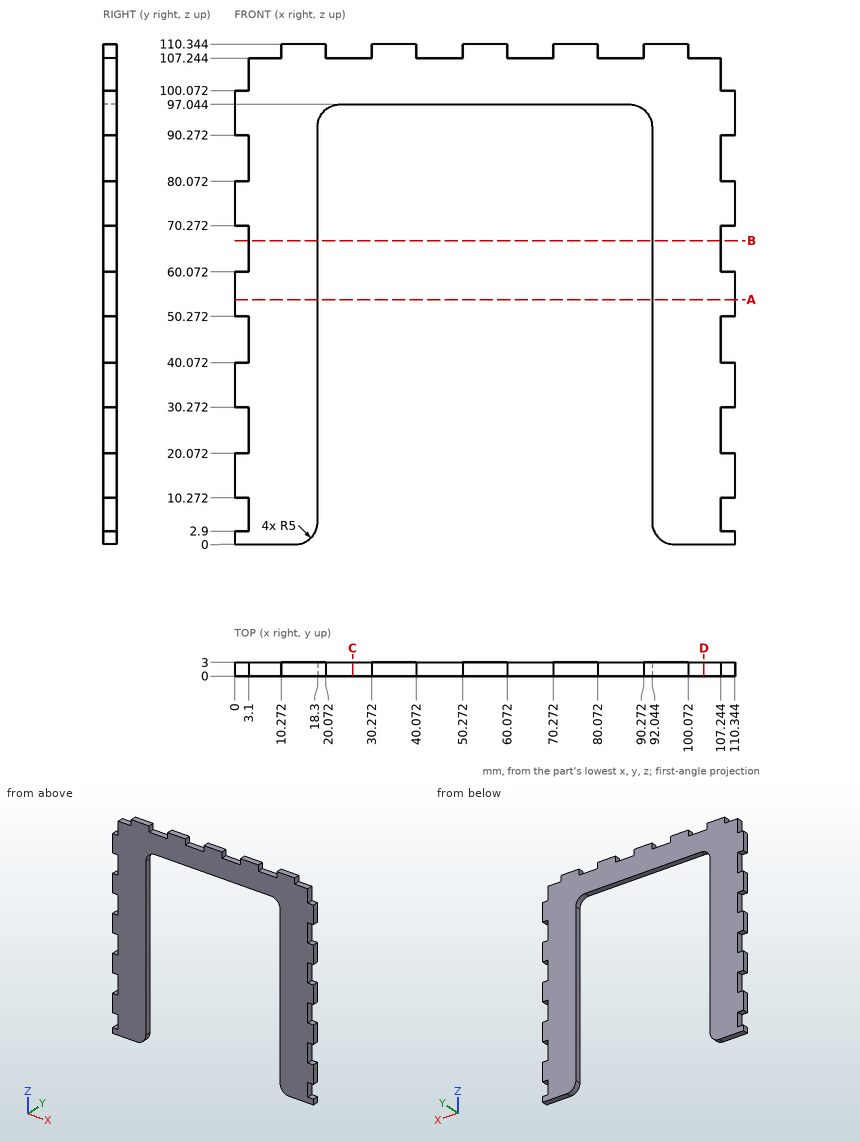
Answer from the drawing. Dimensions are ordinates in mm from the lowest x, y and z of the part. Give positions to 0.01 mm unless a question says otherwise; leave off trailing zeros. Write each loop counter-clockwise with the first axis right and the second up, starting at its lowest first coordinate (ties: lowest second). Pieces come first, ordered by that corner, then holes. Notation, with made-up numbers: (-38, 77) -> (10, 77) arc R8 cw to (10, 92) -> close; hole circle Ø11 at (-28, 48.5). An arc over 180 degrees is marked (long way). Use a Markdown table: item, result.
(1) Flat-ended cylindrical pins translate along their axes: P1, Ø0.9, axis at y = 1, z = 86.5, coming from the -X side; P2, Ø0.9, axis at x = 102, y = 1, coming from the +Z side; P3, Ø0.9, axis at y = 2, z = 7, coming from the +X side. Find the tip coordinate at first contact, or state that the pin passes through.
Return value:
| item | result |
|---|---|
| P1 | x = 3.1 |
| P2 | z = 107.24 |
| P3 | x = 107.24 |
(2) Section C-C, the plane x = 26 is taken. Determine the outline of the cut face in (y, z) (1 decimal), then the cut area to 3 significant figures.
Return value:
| item | result |
|---|---|
| outline | (0, 97) -> (3, 97) -> (3, 107.2) -> (0, 107.2) -> close |
| area | 30.6 mm2 |
(3) Section D-D, the plane x = 103.5 is taken. Determine the outline of the cut face in (y, z) (1 decimal).
Return value:
| item | result |
|---|---|
| outline | (0, 0) -> (3, 0) -> (3, 107.2) -> (0, 107.2) -> close |
(4) Find the intervals of material crossed by probe 1 along X at (y, z) = (0.15, 9.5) (1 decimal); probe 2 along X at (y, z) = (2.6, 78) (1 decimal); probe 3 along Z at (x, y) = (43.5, 2.55) (1 decimal), in increasing order. Write a range as from..to.
Return value:
| item | result |
|---|---|
| probe 1 | 3.1..18.3, 92..107.2 |
| probe 2 | 0..18.3, 92..110.3 |
| probe 3 | 97..107.2 |
(5) Section B-B, the plane z = 67 is taken. Determine the outline of the cut face in (x, y) (1 decimal).
Return value:
| item | result |
|---|---|
| outline | (3.1, 0) -> (18.3, 0) -> (18.3, 3) -> (3.1, 3) -> close; (92, 0) -> (107.2, 0) -> (107.2, 3) -> (92, 3) -> close |
(6) Section A-A, the plane z = 54 is taken. Determine the outline of the cut face in (x, y) (1 decimal), then the cut area to 3 significant figures.
Return value:
| item | result |
|---|---|
| outline | (0, 0) -> (18.3, 0) -> (18.3, 3) -> (0, 3) -> close; (92, 0) -> (110.3, 0) -> (110.3, 3) -> (92, 3) -> close |
| area | 110 mm2 |
